Source: three-view drawing plus pictorial views. Frame: mm from the lowest corner of the part. Round coordinates to 2 decimals unless told otherwise and drop trailing zeros. Loops run counter-clockwise (first coordinate to the right, second up) from the corner with the lowest first, then second, coordinate; pieces in that order, holes last. Notation, with made-up numbers: (19, 73.5) -> (32, 73.5) arc R11 ccw to (32, 83.5) -> close; hole circle Ø1 at (-22.75, -32.75). An arc over 180 degrees is marked (long way). Put each result on its own line as item: value. Start each with the question number.
1. Cut plane A-A (z = 65). Return the cut outline in (x, y).
2. Cut plane B-B (x = 73). Return the cut outline in (y, z), then the cut area to 3 significant figures.
3. Cut plane C-C (y = 2.15). Return the cut outline in (x, z), then the cut area to 3 significant figures.
4. Cut plane D-D (z = 15). Return the cut outline in (x, y).
5. Material intervals for L1, parallel to X at y = 2.6, z = 70; L2, parallel to X at y = 1.7, z = 15; L3, parallel to Z at x = 8, y = 3, sorted ascending.
6. Contact query for flat-ended pins moving along their axis: pin 1 (2.5 mm diameter, centred on y = 2.5, z = 60, fed in from +X); pin 2 (1.5 mm diameter, centred on x = 71.5, y = 3, fed in from +Z); pin 3 (2 mm diameter, centred on y = 2.5, z = 29, fed in from -X). Output: stop coordinate, or through.
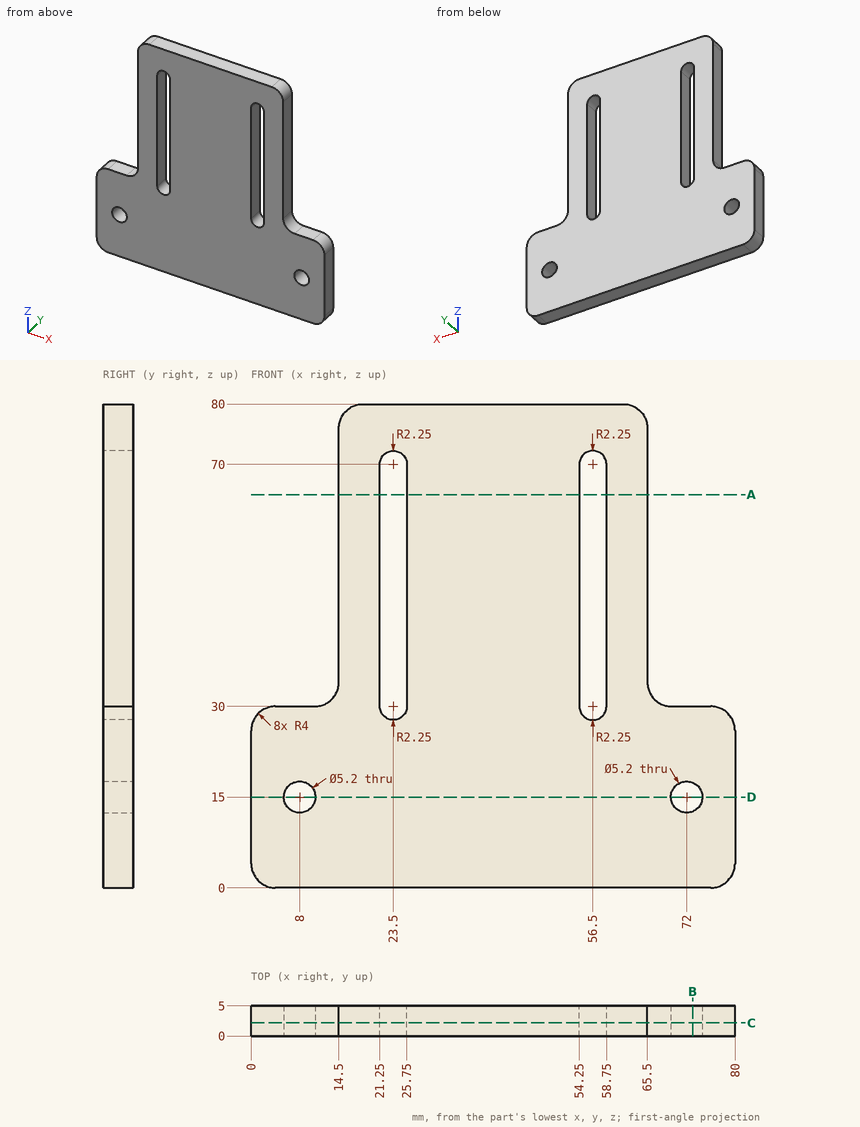
Solution:
1. outline: (14.5, 0) -> (21.25, 0) -> (21.25, 5) -> (14.5, 5) -> close; (25.75, 0) -> (54.25, 0) -> (54.25, 5) -> (25.75, 5) -> close; (58.75, 0) -> (65.5, 0) -> (65.5, 5) -> (58.75, 5) -> close
2. outline: (0, 0) -> (5, 0) -> (5, 12.6) -> (0, 12.6) -> close; (0, 17.4) -> (5, 17.4) -> (5, 30) -> (0, 30) -> close
2. area: 126 mm^2
3. outline: (0, 4) arc R4 ccw to (4, 0) -> (76, 0) arc R4 ccw to (80, 4) -> (80, 26) arc R4 ccw to (76, 30) -> (69.5, 30) arc R4 cw to (65.5, 34) -> (65.5, 76) arc R4 ccw to (61.5, 80) -> (18.5, 80) arc R4 ccw to (14.5, 76) -> (14.5, 34) arc R4 cw to (10.5, 30) -> (4, 30) arc R4 ccw to (0, 26) -> close; hole circle Ø5.2 at (8, 15); hole (21.25, 30) arc R2.25 ccw to (25.75, 30) -> (25.75, 70) arc R2.25 ccw to (21.25, 70) -> close; hole (54.25, 30) arc R2.25 ccw to (58.75, 30) -> (58.75, 70) arc R2.25 ccw to (54.25, 70) -> close; hole circle Ø5.2 at (72, 15)
3. area: 4,500 mm^2
4. outline: (0, 0) -> (5.4, 0) -> (5.4, 5) -> (0, 5) -> close; (10.6, 0) -> (69.4, 0) -> (69.4, 5) -> (10.6, 5) -> close; (74.6, 0) -> (80, 0) -> (80, 5) -> (74.6, 5) -> close
5. L1: x = 14.5 to 21.25, 25.75 to 54.25, 58.75 to 65.5
5. L2: x = 0 to 5.4, 10.6 to 69.4, 74.6 to 80
5. L3: z = 0 to 12.4, 17.6 to 30
6. pin 1: stops at x = 65.5
6. pin 2: stops at z = 30
6. pin 3: stops at x = 0.54
